Source: CAD feature listing. Evaluate the final solid. Frame: model axes, mm. A direction names the side the tool comes from. Give positions to 0.01 mm unless a question says otherwise; leave off trailing zeros. Write each loop counter-clockwise with the first axis right and the second up, starting at its lowest first coordinate (ties: lowest second). Pieces come first, ordered by that corner, then holes. Notation, with made-up numbers: M 25,13 L 36,13 A16 ccw 36,37 Z; hole C 56.5,-7 d10. An arc over 180 degrees is marked long. Return JSON: item names as keys, results as strings.
```python
from build123d import *

# Parameters (mm, degrees)
SKETCH_1_W           = 50
SKETCH_1_H           = 13
EXTRUDE_1_DEPTH      = 48
SKETCH_9_R           = 1.6
CUT_EXTRUDE_7_DEPTH  = 14
SKETCH_10_R          = 3
CUT_EXTRUDE_10_DEPTH = 3.6
SKETCH_2_W           = 4
SKETCH_2_H           = 6
CUT_EXTRUDE_15_DEPTH = 51
SKETCH_18_W          = 20
SKETCH_18_H          = 7
CUT_EXTRUDE_16_DEPTH = 51
SKETCH_19_W          = 13
SKETCH_19_H          = 1
CUT_EXTRUDE_17_DEPTH = 51
SKETCH_21_W          = 8
SKETCH_21_H          = 6
CUT_EXTRUDE_19_DEPTH = 51
CHAMFER_1_SIZE       = 2
CUT_EXTRUDE_START    = 8
SKETCH_22_W          = 10
SKETCH_22_H          = 9
CUT_EXTRUDE_20_DEPTH = 49
CHAMFER_2_SIZE       = 3
CHAMFER_2_SIZE2      = 1.94822278
SKETCH_23_W          = 9
SKETCH_23_H          = 2.5
CUT_EXTRUDE_21_DEPTH = 41
SKETCH_26_W          = 7
SKETCH_26_H          = 4
CUT_EXTRUDE_24_DEPTH = 49
SKETCH_27_W          = 4
SKETCH_27_H          = 7
EXTRUDE_2_DEPTH      = 5
SKETCH_37_R          = 1.25
CUT_EXTRUDE_30_DEPTH = 5
SKETCH_38_W          = 15
SKETCH_38_H          = 8
EXTRUDE_3_DEPTH      = 17
SKETCH_39_W          = 10.2
SKETCH_39_H          = 21.5
CUT_EXTRUDE_31_DEPTH = 1.3
FILLET_2_R           = 1
SKETCH_40_R          = 1.25
CUT_EXTRUDE_32_DEPTH = 6
SKETCH_41_W          = 7
SKETCH_41_H          = 22
CUT_EXTRUDE_33_DEPTH = 4
SKETCH_43_W          = 7
SKETCH_43_H          = 12
CUT_EXTRUDE_35_DEPTH = 8
FILLET_3_R           = 1
SKETCH_44_W          = 19.428817274
SKETCH_44_H          = 15
CUT_EXTRUDE_37_DEPTH = 8
SKETCH_45_R          = 1.25
CUT_EXTRUDE_38_DEPTH = 5.5
SKETCH_46_W          = 45.087872193
SKETCH_46_H          = 5.805305433
CUT_EXTRUDE_39_DEPTH = 9


with BuildPart() as part:
    # Эскиз1 → Бобышка-Вытянуть1 (new body)
    with BuildSketch(Plane.XY):
        Rectangle(SKETCH_1_W, SKETCH_1_H)
    extrude(amount=EXTRUDE_1_DEPTH)

    # Эскиз9 → Вырез-Вытянуть7 (cut, through all)
    with BuildSketch(Plane(origin=(0, 6.5, 0), x_dir=(1, 0, 0), z_dir=(0, 1, 0))):
        with Locations(Location((20, -41.5, 0), (0, 0, 270))):  # turned: the seam where the file's is
            Circle(SKETCH_9_R)
        with Locations(Location((10, -41.5, 0), (0, 0, 270))):  # turned: the seam where the file's is
            Circle(SKETCH_9_R)
        with Locations(Location((0, -41.5, 0), (0, 0, 270))):  # turned: the seam where the file's is
            Circle(SKETCH_9_R)
    extrude(amount=-CUT_EXTRUDE_7_DEPTH, mode=Mode.SUBTRACT)

    # Эскиз10 → Вырез-Вытянуть10 (cut)
    with BuildSketch(Plane(origin=(0, 6.5, 0), x_dir=(1, 0, 0), z_dir=(0, 1, 0))):
        with Locations(Location((20, -41.5, 0), (0, 0, 270))):  # turned: the seam where the file's is
            Circle(SKETCH_10_R)
        with Locations(Location((10, -41.5, 0), (0, 0, 270))):  # turned: the seam where the file's is
            Circle(SKETCH_10_R)
        with Locations(Location((0, -41.5, 0), (0, 0, 270))):  # turned: the seam where the file's is
            Circle(SKETCH_10_R)
    extrude(amount=-CUT_EXTRUDE_10_DEPTH, mode=Mode.SUBTRACT)

    # Эскиз2 → Вырез-Вытянуть15 (cut, through all)
    with BuildSketch(Plane.ZY.offset(25)):
        with Locations((46, -3.5)):
            Rectangle(SKETCH_2_W, SKETCH_2_H)
    extrude(amount=-CUT_EXTRUDE_15_DEPTH, mode=Mode.SUBTRACT)

    # Эскиз18 → Вырез-Вытянуть16 (cut, through all)
    with BuildSketch(Plane.ZY.offset(25)):
        with Locations((23, -3)):
            Rectangle(SKETCH_18_W, SKETCH_18_H)
    extrude(amount=-CUT_EXTRUDE_16_DEPTH, mode=Mode.SUBTRACT)

    # Эскиз19 → Вырез-Вытянуть17 (cut, through all)
    with BuildSketch(Plane(origin=(25, 0, 0), x_dir=(0, 0, -1), z_dir=(1, 0, 0))):
        with Locations((-6.5, -6)):
            Rectangle(SKETCH_19_W, SKETCH_19_H)
    extrude(amount=-CUT_EXTRUDE_17_DEPTH, mode=Mode.SUBTRACT)

    # Эскиз21 → Вырез-Вытянуть19 (cut, through all)
    with BuildSketch(Plane(origin=(25, 0, 0), x_dir=(0, 0, -1), z_dir=(1, 0, 0))):
        with Locations((-4, -2.5)):
            Rectangle(SKETCH_21_W, SKETCH_21_H)
    extrude(amount=-CUT_EXTRUDE_19_DEPTH, mode=Mode.SUBTRACT)

    # Фаска1
    chamfer_1_edges = [part.edges().sort_by_distance(p)[0] for p in [
        (0, 0.5, 0),
    ]]
    chamfer(chamfer_1_edges, length=CHAMFER_1_SIZE)

    # Эскиз22 → Вырез-Вытянуть20 (cut, through all)
    with BuildSketch(Plane(origin=(0, 0, 8), x_dir=(-1, 0, 0), z_dir=(0, 0, -1)).offset(CUT_EXTRUDE_START)):
        with Locations((20, -2)):
            Rectangle(SKETCH_22_W, SKETCH_22_H)
    extrude(amount=-CUT_EXTRUDE_20_DEPTH, mode=Mode.SUBTRACT)

    # Фаска2
    chamfer_2_edges = [part.edges().sort_by_distance(p)[0] for p in [
        (-15, 2.5, 24),
    ]]
    chamfer_2_side = [part.faces().sort_by_distance(p)[0] for p in [
        (-20, 2.5, 24),
    ]]
    chamfer(chamfer_2_edges, length=CHAMFER_2_SIZE, length2=CHAMFER_2_SIZE2, reference=chamfer_2_side[0])

    # Эскиз23 → Вырез-Вытянуть21 (cut, through all)
    with BuildSketch(Plane(origin=(0, 0, 8), x_dir=(-1, 0, 0), z_dir=(0, 0, -1))):
        with Locations((10.5, -0.75)):
            Rectangle(SKETCH_23_W, SKETCH_23_H)
    extrude(amount=-CUT_EXTRUDE_21_DEPTH, mode=Mode.SUBTRACT)

    # Эскиз26 → Вырез-Вытянуть24 (cut, through all)
    with BuildSketch(Plane(origin=(0, 0, 0), x_dir=(-1, 0, 0), z_dir=(0, 0, -1))):
        with Locations((21.5, 4.5)):
            Rectangle(SKETCH_26_W, SKETCH_26_H)
    extrude(amount=-CUT_EXTRUDE_24_DEPTH, mode=Mode.SUBTRACT)

    # Эскиз27 → Бобышка-Вытянуть2 (add)
    with BuildSketch(Plane.ZY.offset(18)):
        with Locations((46, 3)):
            Rectangle(SKETCH_27_W, SKETCH_27_H)
    extrude(amount=-EXTRUDE_2_DEPTH)

    # Эскиз37 → Вырез-Вытянуть30 (cut)
    with BuildSketch(Plane(origin=(0, 6.5, 0), x_dir=(1, 0, 0), z_dir=(0, 1, 0))):
        with Locations(Location((10, -34.5, 0), (0, 0, 270))):  # turned: the seam where the file's is
            Circle(SKETCH_37_R)
        with Locations(Location((10, -11.5, 0), (0, 0, 270))):  # turned: the seam where the file's is
            Circle(SKETCH_37_R)
    extrude(amount=-CUT_EXTRUDE_30_DEPTH, mode=Mode.SUBTRACT)

    # Эскиз38 → Бобышка-Вытянуть3 (add)
    with BuildSketch(Plane(origin=(0, 6.5, 0), x_dir=(1, 0, 0), z_dir=(0, 1, 0))):
        with Locations((-10.5, -44)):
            Rectangle(SKETCH_38_W, SKETCH_38_H)
    extrude(amount=EXTRUDE_3_DEPTH)

    # Эскиз39 → Вырез-Вытянуть31 (cut)
    with BuildSketch(Plane.XY.offset(48)):
        with Locations((-9.65, 10.25)):
            Rectangle(SKETCH_39_W, SKETCH_39_H)
    extrude(amount=-CUT_EXTRUDE_31_DEPTH, mode=Mode.SUBTRACT)

    # Скругление2
    fillet_2_edges = [part.edges().sort_by_distance(p)[0] for p in [
        (-14.75, 21, 47.35),
        (-4.55, 21, 47.35),
    ]]
    fillet(fillet_2_edges, radius=FILLET_2_R)

    # Эскиз40 → Вырез-Вытянуть32 (cut)
    with BuildSketch(Plane.XY.offset(46.7)):
        with Locations((-9.65, 8.9)):
            Circle(SKETCH_40_R)
    extrude(amount=-CUT_EXTRUDE_32_DEPTH, mode=Mode.SUBTRACT)

    # Эскиз41 → Вырез-Вытянуть33 (cut)
    with BuildSketch(Plane.XY.offset(46.7)):
        with Locations((-9.65, 4.5)):
            Rectangle(SKETCH_41_W, SKETCH_41_H)
    extrude(amount=-CUT_EXTRUDE_33_DEPTH, mode=Mode.SUBTRACT)

    # Эскиз43 → Вырез-Вытянуть35 (cut)
    with BuildSketch(Plane.XY.offset(42.7)):
        with Locations((-9.65, -0.5)):
            Rectangle(SKETCH_43_W, SKETCH_43_H)
    extrude(amount=-CUT_EXTRUDE_35_DEPTH, mode=Mode.SUBTRACT)

    # Скругление3
    fillet_3_edges = [part.edges().sort_by_distance(p)[0] for p in [
        (-6.15, 15.5, 44.7),
        (-13.15, 15.5, 44.7),
    ]]
    fillet(fillet_3_edges, radius=FILLET_3_R)

    # Эскиз44 → Вырез-Вытянуть37 (cut)
    with BuildSketch(Plane(origin=(0, 6.5, 0), x_dir=(1, 0, 0), z_dir=(0, 1, 0))):
        with Locations((-8.285591363, -23)):
            Rectangle(SKETCH_44_W, SKETCH_44_H)
    extrude(amount=-CUT_EXTRUDE_37_DEPTH, mode=Mode.SUBTRACT)

    # Эскиз45 → Вырез-Вытянуть38 (cut)
    with BuildSketch(Plane(origin=(0, 6.5, 0), x_dir=(1, 0, 0), z_dir=(0, 1, 0))):
        with Locations(Location((-9.75, -5, 0), (0, 0, 270))):  # turned: the seam where the file's is
            Circle(SKETCH_45_R)
    extrude(amount=-CUT_EXTRUDE_38_DEPTH, mode=Mode.SUBTRACT)

    # Эскиз46 → Вырез-Вытянуть39 (cut)
    with BuildSketch(Plane.ZY.offset(15)):
        with Locations((23.854867364, -4.199105634)):
            Rectangle(SKETCH_46_W, SKETCH_46_H)
    extrude(amount=-CUT_EXTRUDE_39_DEPTH, mode=Mode.SUBTRACT)


solid = part.part
```
1) Draft query along X for faces 1 (the face through (10, 1.5, 34)), 2 (the face through (1.429, 4, 23)), 3 (the face through (-8, 4, 15.5)). Return one class per face: released by +X, released by -X, zero draft, split by the parting line, or undercut.
Numbers:
{"face 1": "undercut", "face 2": "released by -X", "face 3": "zero draft"}
2) Cut plane C-C, the plane y = 4. Return the cut outline in (x, z).
Numbers:
{"outline": "M -18,0 L 25,0 L 25,48 L -4.55,48 L -4.55,46.7 L -6.15,46.7 L -6.15,34.7 L -13.15,34.7 L -13.15,46.7 L -14.75,46.7 L -14.75,48 L -18,48 L -18,30.5 L 1.43,30.5 L 1.43,15.5 L -18,15.5 Z; hole C -9.75,5 d2.5; hole C 0,41.5 d6; hole C 10,41.5 d6; hole C 10,11.5 d2.5; hole C 10,34.5 d2.5; hole C 20,41.5 d6"}
3) Line query: line 1 (Z direction, x = 0, y = 5.3); line 2 (Z direction, x = 18, y = -3.75); line 3 (X direction, y = 4.7, z = 41.5). Output: solid intervals per line, ascending. Write a range as [from, to].
Numbers:
{"line 1": "z = [0, 15.5], [30.5, 38.5], [44.5, 48]", "line 2": "z = [8, 13], [33, 44]", "line 3": "x = [-18, -13.15], [-6.15, -3], [3, 7], [13, 17], [23, 25]"}
4) Cut plane D-D, the plane z = 7. Return the cut outline in (x, y).
Numbers:
{"outline": "M -18,2.5 L -15,0.55 L -15,0.5 L 25,0.5 L 25,6.5 L -18,6.5 Z"}
5) Set-up query: faces 4 (the face through (10, 1.5, 11)), 5 (the face through (-14.75, 10, 47)), 6 (the face through (9, -3, 33)). Return all of +Z, -Z, +X, -X, +Y, -Y with unobstructed straight access to the full face (end or side cutting, diameter ignored); none if empty.
Numbers:
{"face 4": "+Y", "face 5": "+Z, -Y", "face 6": "+X, -X, -Y"}
6) Cut plane B-B, the plane y = -3.5. Return the cut outline in (x, z).
Numbers:
{"outline": "M -6,8 L 25,8 L 25,13 L -6,13 Z; M -6,33 L 25,33 L 25,44 L -6,44 Z; hole C 0,41.5 d3.2; hole C 10,41.5 d3.2; hole C 20,41.5 d3.2"}
7) Contact query for flat-ended pins moving along their axis: pin 1 Ø2 at (x, z) = (10, 11.5) entering from +Y; pin 2 Ø5 at (x, z) = (0, 9.5) entering from -Y; pin 3 Ø0.6 at (y, z) = (9, 47) entering from +X; pin 4 Ø8 at (x, z) = (-8.5, 22.5) entering from +Y. Output: stop coordinate, or through.
Numbers:
{"pin 1": "stops at y = 1.5", "pin 2": "stops at y = -5.5", "pin 3": "stops at x = -3", "pin 4": "passes through"}
